For this review, use the dimensioned drawing (mm, ordinates from the lowest corner) and the shaded views. Coordinates: 2 decimals unless noted, no trailing zeros. Write each loop counter-clockwise with the first axis right and the second up, starting at its lowest first coordinate (ties: lowest second). Pieces come first, ordered by that corner, then holes. Notation, with made-up numbers: (9.5, -14) - (13.5, -14) arc R22 ccw to (13.5, 4) - close; hole circle Ø3 at (-16.75, -21). An arc over 180 degrees is marked (long way). One line per item, written item: value.
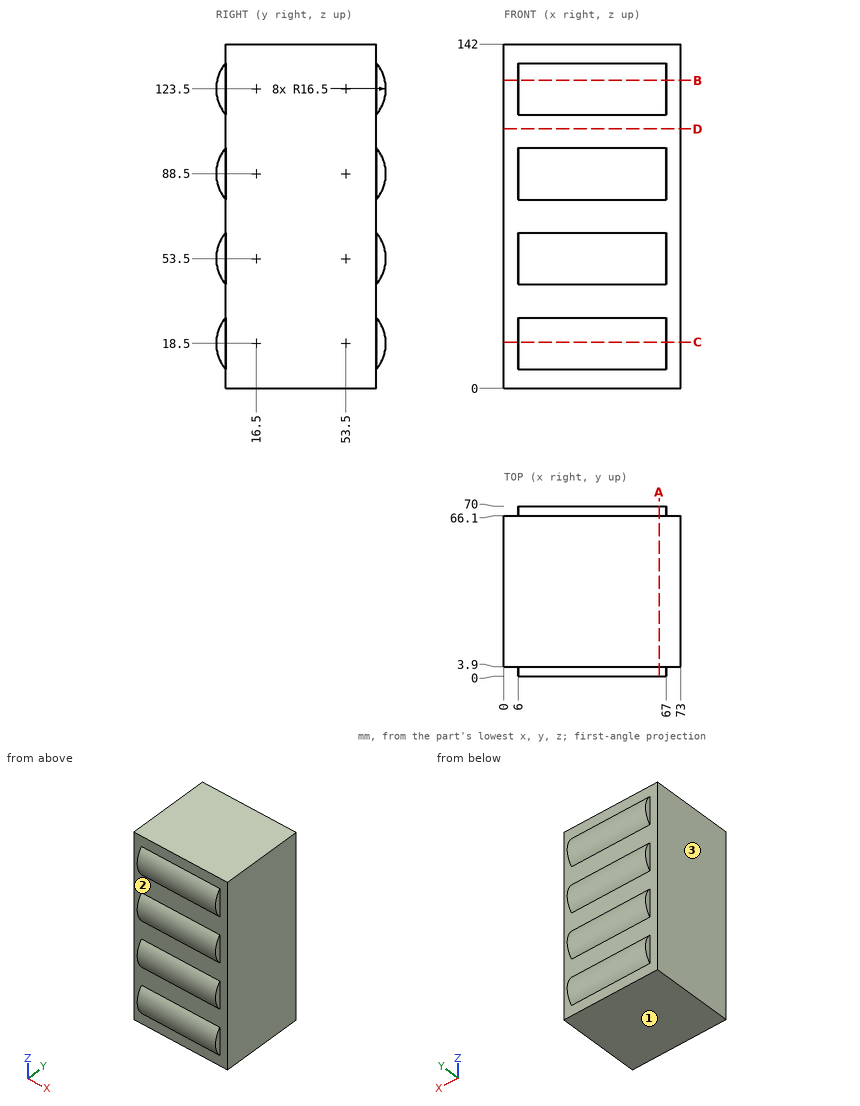
1. Wall thickness on line 1 along Z through (x, y) = (19, 66.5); line 2 along Y through (x, z) = (48, 110); line 3 along Y through (x, z) = (36, 43): over which ranges is each line inside the solid? List them lowest first.
Answer block:
line 1: z = 8.34 to 28.66, 43.34 to 63.66, 78.34 to 98.66, 113.34 to 133.66
line 2: y = 3.9 to 66.1
line 3: y = 3.77 to 66.23
2. Mouldability with a two-part tool opening along Z and no side actions: class the marked faces 1, 2 and 3 as released by +Z, released by -Z, zero draft, split by the parting line, or undercut.
Answer block:
face 1: released by -Z
face 2: undercut
face 3: zero draft
3. Consider section D-D, the plane z = 107. Write out the cut boundary in (x, y).
Answer block:
outline: (0, 3.9) - (73, 3.9) - (73, 66.1) - (0, 66.1) - close
4. Consider section C-C, the plane z = 19. Write out the cut boundary in (x, y), then the cut area to 3 significant figures.
Answer block:
outline: (0, 3.9) - (6, 3.9) - (6, 0.01) - (67, 0.01) - (67, 3.9) - (73, 3.9) - (73, 66.1) - (67, 66.1) - (67, 69.99) - (6, 69.99) - (6, 66.1) - (0, 66.1) - close
area: 5,020 mm^2
5. Consider section A-A, the plane x = 64. Write out the cut boundary in (y, z), then the cut area to 3 significant figures.
Answer block:
outline: (3.9, 0) - (66.1, 0) - (66.1, 7.85) arc R16.5 ccw to (66.1, 29.15) - (66.1, 42.85) arc R16.5 ccw to (66.1, 64.15) - (66.1, 77.85) arc R16.5 ccw to (66.1, 99.15) - (66.1, 112.85) arc R16.5 ccw to (66.1, 134.15) - (66.1, 142) - (3.9, 142) - (3.9, 134.15) arc R16.5 ccw to (3.9, 112.85) - (3.9, 99.15) arc R16.5 ccw to (3.9, 77.85) - (3.9, 64.15) arc R16.5 ccw to (3.9, 42.85) - (3.9, 29.15) arc R16.5 ccw to (3.9, 7.85) - close
area: 9,290 mm^2
6. Insertion check: pin 1 Ø3 at (y, z) = (1.5, 16.5) entering from +X; pin 2 Ø4 at (x, z) = (9, 85.5) entering from -Y; pin 3 Ø1.5 at (x, z) = (44.5, 31.5) entering from +Y. Each pin has a flat end and moves straight along its axis. Give the tip position at first contact, or say it passes through.
Answer block:
pin 1: stops at x = 67
pin 2: stops at y = 0.03
pin 3: stops at y = 66.1
7. Consider section B-B, the plane z = 127. Write out the cut boundary in (x, y), then the cut area to 3 significant figures.
Answer block:
outline: (0, 3.9) - (6, 3.9) - (6, 0.38) - (67, 0.38) - (67, 3.9) - (73, 3.9) - (73, 66.1) - (67, 66.1) - (67, 69.62) - (6, 69.62) - (6, 66.1) - (0, 66.1) - close
area: 4,970 mm^2
